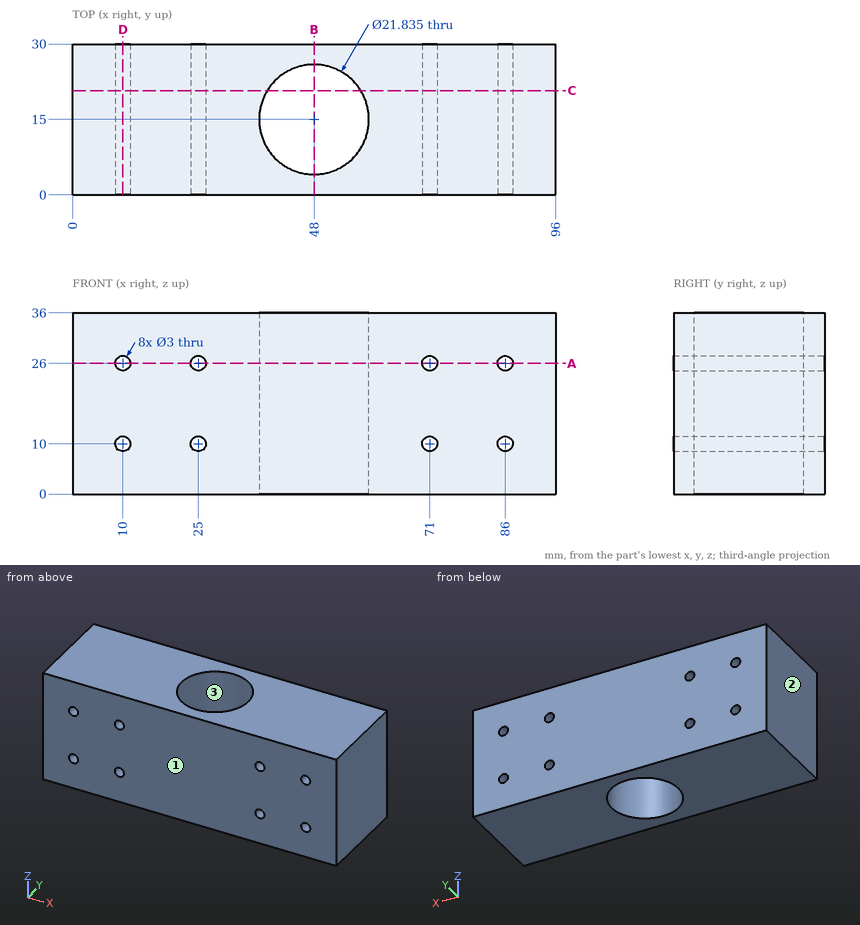
Geometry check sheet. Reference: drawing and pictorial views, mm from the part's lowest x, y, z. Round coordinates to 2 decimals unless told otherwise and drop trailing zeros. Loops run counter-clockwise (first coordinate to the right, second up) from the corner with the lowest first, then second, coordinate; pieces in that order, holes last. Notation, with made-up numbers: M -23.75,44 L -15.75,44 A15 ccw -15.75,51 Z; hole C 60.25,67.25 d4. An arc over 180 degrees is marked long. One line per item, written item: value.
(1) Depth check by flat-ended pin: pin 1 Ø4 at (x, z) = (25, 26) entering from +Y; pin 2 Ø2.5 at (x, z) = (71, 10) entering from -Y. Enter the tip coordinate at first touch or a pass-through.
Computed values:
pin 1: stops at y = 30
pin 2: passes through
(2) Thickness scan on line 1 (Z direction, x = 86, y = 11); line 2 (X direction, y = 8.5, z = 10); line 3 (X direction, y = 24.25, z = 10). Record the ranges inside material, lowest first.
Computed values:
line 1: z = 0 to 8.5, 11.5 to 24.5, 27.5 to 36
line 2: x = 0 to 8.5, 11.5 to 23.5, 26.5 to 39.23, 56.77 to 69.5, 72.5 to 84.5, 87.5 to 96
line 3: x = 0 to 8.5, 11.5 to 23.5, 26.5 to 42.2, 53.8 to 69.5, 72.5 to 84.5, 87.5 to 96
(3) Release check for a two-part mould opening along X. For the marked faces 1, 2 and 3 record: +X half, -X half, draft (parallel to the pull), parting line (faces both ways), or undercut.
Computed values:
face 1: draft
face 2: -X half
face 3: undercut
(4) Sectioned sample at B-B, the plane x = 48. Record the cut outline in (y, z).
Computed values:
outline: M 0,0 L 4.08,0 L 4.08,36 L 0,36 Z; M 25.92,0 L 30,0 L 30,36 L 25.92,36 Z
(5) Sectioned sample at C-C, the plane y = 20.75. Count the separate pieces of the cut face and the enclosed holes in it, then the cut area to 3 significant figures.
Computed values:
separate pieces: 2
enclosed holes: 8
area: 2,730 mm^2
(6) Sectioned sample at A-A, the plane z = 26. Record the cut outline in (x, y) (1 decimal).
Computed values:
outline: M 0,0 L 8.5,0 L 8.5,30 L 0,30 Z; M 11.5,0 L 23.5,0 L 23.5,30 L 11.5,30 Z; M 26.5,0 L 69.5,0 L 69.5,30 L 26.5,30 Z; M 72.5,0 L 84.5,0 L 84.5,30 L 72.5,30 Z; M 87.5,0 L 96,0 L 96,30 L 87.5,30 Z; hole C 48,15 d21.8
(7) Sectioned sample at D-D, the plane x = 10. Record the cut outline in (y, z).
Computed values:
outline: M 0,0 L 30,0 L 30,8.5 L 0,8.5 Z; M 0,11.5 L 30,11.5 L 30,24.5 L 0,24.5 Z; M 0,27.5 L 30,27.5 L 30,36 L 0,36 Z
